from build123d import *

# Parameters (mm, degrees)
SKETCH1_R           = 15.25
BOSS_EXTRUDE1_DEPTH = 23.5
SKETCH2_R           = 5
BOSS_EXTRUDE2_DEPTH = 2.25
SHELL1_T            = -0.5
SKETCH3_R           = 1.75
CUT_EXTRUDE1_DEPTH  = 4.5


with BuildPart() as part:
    # Sketch1 → Boss-Extrude1 (new, symmetric)
    with BuildSketch(Plane.XY):
        Circle(SKETCH1_R)
    extrude(amount=BOSS_EXTRUDE1_DEPTH, both=True)

    # Sketch2 → Boss-Extrude2 (add, symmetric)
    with BuildSketch(Plane.XY.offset(23.5)):
        Circle(SKETCH2_R)
    extrude(amount=BOSS_EXTRUDE2_DEPTH, both=True)

    # Shell1
    shell1_openings = [part.faces().sort_by_distance(p)[0] for p in [
        (0, 0, -23.5),
        (0, 0, 25.75),
    ]]
    offset(amount=SHELL1_T, openings=shell1_openings, kind=Kind.INTERSECTION)

    # Sketch3 → Cut-Extrude1 (cut)
    with BuildSketch(Plane.XY.offset(23.5)):
        with Locations((-10, 0)):
            Circle(SKETCH3_R)
        with Locations((0, 10)):
            Circle(SKETCH3_R)
        with Locations((10, 0)):
            Circle(SKETCH3_R)
    extrude(amount=-CUT_EXTRUDE1_DEPTH, mode=Mode.SUBTRACT)


solid = part.part
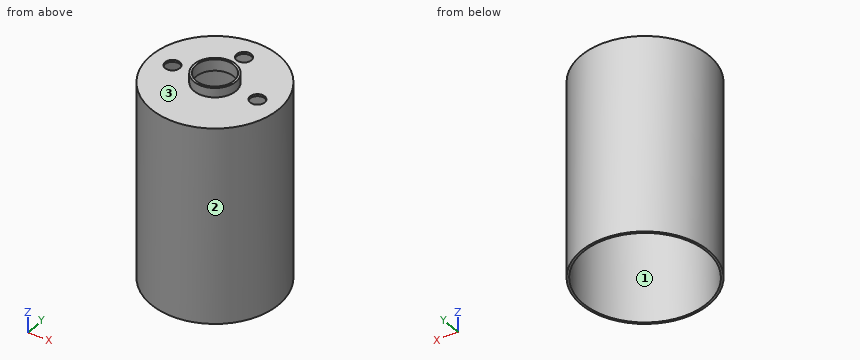
Here's how the part is built. I have some questions about the finished solid (model axes, mm). Face numbers are marked on the shaded views. Give positions to 0.01 mm unless a question says otherwise; leave off trailing zeros. Order: outer loops, then holes, each group sorted by start corner. A loop starts at its lowest first (then second) coordinate and runs counter-clockwise, first axis right, second up. Notation, with made-up numbers: M 35.25,73 L 84.25,73 A18 cw 84.25,95 Z; hole C -16,39.5 d4. An arc over 180 degrees is marked long. Answer as a JSON object with one key per item and string values. Group by question number.
1) Suppose I cut it at A-A, the plane x = 0. Write out the boundary of the cut face in (y, z).
2) Suppose I cut it at C-C, the plane x = -10. Write out the boundary of the cut face in (y, z), plus the area to 3 significant figures.
3) Suppose I cut it at B-B, the plane y = -3.5. Write out the boundary of the cut face in (x, z), plus the area to 3 significant figures.
4) We'd pull the mould along X, two halves only. Please class the marked faces 1, 2 and 3: pulls with the +X half, pulls with the -X half, needs draft (parallel to the pull), parting line crosses it, or undercut.
5) I'm going to push flat-ended pins straight in: pin 1 Ø6 at (x, z) = (5, 13.5) entering from -Y; pin 2 Ø2 at (x, y) = (6, 0.5) entering from -Z; pin 3 Ø5 at (y, z) = (-9, -2.5) entering from +X. Where does each tip first touch, or does it pass through?
6) Suppose I cut it at D-D, the plane z = -10. Write out the boundary of the cut face in (x, y).
7) Please list where these lines run through material, in increasing order: L1, parallel to Y at x = 0, z = -2; L2, parallel to Z at x = -4, y = -13.5; L3, parallel to X at y = -1, z = -21. Write a range as [from, to].
Results found:
{
 "1": {"outline": "M -15.25,-23.5 L -14.75,-23.5 L -14.75,23 L -4.5,23 L -4.5,25.75 L -5,25.75 L -5,23.5 L -15.25,23.5 Z; M 4.5,23 L 8.25,23 L 8.25,23.5 L 5,23.5 L 5,25.75 L 4.5,25.75 Z; M 11.75,23 L 14.75,23 L 14.75,-23.5 L 15.25,-23.5 L 15.25,23.5 L 11.75,23.5 Z"},
 "2": {"outline": "M -11.51,-23.5 L -10.84,-23.5 L -10.84,23 L -1.75,23 L -1.75,23.5 L -11.51,23.5 Z; M 1.75,23 L 10.84,23 L 10.84,-23.5 L 11.51,-23.5 L 11.51,23.5 L 1.75,23.5 Z", "area": "72.2 mm²"},
 "3": {"outline": "M -14.84,-23.5 L -14.33,-23.5 L -14.33,23 L -2.83,23 L -2.83,25.75 L -3.57,25.75 L -3.57,23.5 L -14.84,23.5 Z; M 2.83,23 L 14.33,23 L 14.33,-23.5 L 14.84,-23.5 L 14.84,23.5 L 3.57,23.5 L 3.57,25.75 L 2.83,25.75 Z", "area": "63.2 mm²"},
 "4": {"face 1": "undercut", "face 2": "parting line crosses it", "face 3": "needs draft"},
 "5": {"pin 1": "y = -15.12", "pin 2": "z = 23", "pin 3": "x = 13.8"},
 "6": {"outline": "C 0,0 d30.5; hole C 0,0 d29.5"},
 "7": {"L1": "[-15.25, -14.75], [14.75, 15.25]", "L2": "[23, 23.5]", "L3": "[-15.22, -14.72], [14.72, 15.22]"}
}
